The model under review builds one solid part; all positions refer to its coordinate system, in mm. Face numbers are marked on the shaded views. Coordinates: 2 decimals unless noted, no trailing zeros. Order: outer loops, then holes, each group sorted by start corner. A loop starts at its lowest first (then second) coordinate and runs counter-clockwise, first axis right, second up. Notation, with made-up numbers: M 22.25,-3 L 62.25,-3 A30 ccw 62.25,19 Z; hole C 17,85 d8. An arc over 180 degrees is marked long. Answer as CSV lines item,"result". Start each with the question number.
Q1. Consider section D-D on x = 27.75. Write out the cut boundary in (y, z).
Q2. Consider section C-C on x = 4.25. Write out the cut boundary in (y, z), and give its area (3 significant figures).
Q3. For P1, Ø1, axis at x = 12.5, z = 25.5, coming from the -Y side; P2, Ø3, axis at x = 14.5, y = 26, coming from the +Z side; P3, Ø12, axis at x = 22, y = 1.5, coming from the +Z side, all flat-tipped, find the tip position at first contact; note any pin that passes through.
Q4. Consider section A-A on z = 0. Write out the cut boundary in (x, y).
Q5. Wall thickness on L1, parallel to Z at x = 8.25, y = 0; L2, parallel to Y at x = 12.75, z = -15; L3, parallel to Y at x = 2.5, z = -29: over which ranges is each line inside the solid? List them lowest first. Write a range as [from, to].
Q6. The part is to be moulded in two halves that separate along Y. For the marked faces 1, 2 and 3, say which applies: +Y half, -Y half, draft (parallel to the pull), parting line (faces both ways), or undercut.
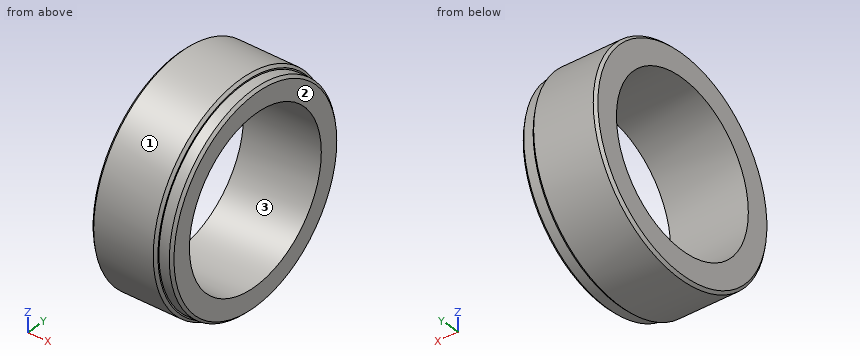
Autodesk Fusion 360 part; units mm, degrees
sketch "Sketch1" plane through (0, 0, 0) normal (1, 0, 0) x (0, 1, 0)
  circle A0 centre (0, 0) radius 42
  circle A1 centre (0, 0) radius 32
  dimension "d1" = 84
  dimension "d2" = 64
extrude "Extrude1" add sketch "Sketch1" along normal blind 25
sketch "Sketch2" plane through (25, 0, 0) normal (1, 0, 0) x (0, 1, 0)
  circle A0 centre (0, 0) radius 32
  circle A1 centre (0, 0) radius 42
  circle A2 centre (0, 0) radius 32
  circle A3 centre (0, 0) radius 40.5
  dimension "d5" = 8.5
extrude "Extrude2" add sketch "Sketch2" along normal blind 5 contours A3
chamfer "Chamfer1" distance 1 angle 45 3 edges at (0, -39.1577, -15.1878) (25, -39.1577, -15.1878) (30, -37.7593, -14.6454) measured on face at (8.3333, 41.7913, -4.1818) measured on face at (25, 11.2341, 39.8428) measured on face at (30, 37.3967, -3.6019)
Evaluation:
1,outline,"C 0,0 d81; hole C 0,0 d64"
2,outline,"C 0,0 d84; hole C 0,0 d64"
2,area,"2,320 mm²"
3,P1,"stops at y = -33.75"
3,P2,"stops at z = 34.11"
3,P3,"stops at z = 42"
4,outline,"M 0,-41 L 1,-42 L 24,-42 L 25,-41 L 25,-40.5 L 29,-40.5 L 30,-39.5 L 30,-32 L 0,-32 Z; M 0,32 L 30,32 L 30,39.5 L 29,40.5 L 25,40.5 L 25,41 L 24,42 L 1,42 L 0,41 Z"
5,L1,"z = [-42, -32], [32, 42]"
5,L2,"y = [-39.23, -28.27], [28.27, 39.23]"
5,L3,"y = [-30.38, -13.53], [13.53, 30.38]"
6,face 1,"parting line"
6,face 2,"draft"
6,face 3,"undercut"
